from build123d import *

# Parameters (mm, degrees)
BOSS_EXTRUDE1_DEPTH             = 17.5
BOSS_EXTRUDE1_DEPTH_BACK        = 17.5
BOSS_EXTRUDE2_DEPTH             = 16
BOSS_EXTRUDE2_DEPTH_BACK        = 16
SKETCH1_3_R                     = 1
SKETCH1_3_W                     = 27.956190476
SKETCH1_3_H                     = 2.76
BOSS_EXTRUDE3_DEPTH             = 18.625
BOSS_EXTRUDE3_DEPTH_BACK        = 18.625
TAP_DRILL_FOR_2_HELICOIL1_D     = 2.38252
TAP_DRILL_FOR_2_HELICOIL1_DEPTH = 5
TAP_DRILL_FOR_2_HELICOIL1_TIP   = 0.715781221
SKETCH6_R                       = 9.6
SKETCH6_R_2                     = 4
CUT_EXTRUDE1_DEPTH              = 0.5


with BuildPart() as part:
    # Sketch1 → Boss-Extrude1 (new, two sides: drawn at the far end of the back side and taken through both)
    with BuildSketch(Plane.XY.offset(-BOSS_EXTRUDE1_DEPTH_BACK)):
        with BuildLine():
            Line((22.61, 0), (-0.726109068, 0))
            ThreePointArc((-0.726109068, 0), (-1.941229139, -5.326939839), (-5.346190476, -9.6))
            Line((-5.346190476, -9.6), (22.61, -9.6))
            Line((22.61, -9.6), (22.61, 0))
        make_face()
        with BuildLine():
            Line((22.61, 9.6), (-5.346190476, 9.6))
            ThreePointArc((-5.346190476, 9.6), (-1.941229139, 5.326939839), (-0.726109068, 0))
            Line((-0.726109068, 0), (22.61, 0))
            Line((22.61, 0), (22.61, 9.6))
        make_face()
    extrude(amount=BOSS_EXTRUDE1_DEPTH + BOSS_EXTRUDE1_DEPTH_BACK)

    # Sketch1<3> → Boss-Extrude2 (add, two sides: drawn at the far end of the back side and taken through both)
    # profile 1 of 7: a face of its own
    with BuildSketch(Plane.XY.offset(-BOSS_EXTRUDE2_DEPTH_BACK)):
        with BuildLine():
            ThreePointArc((-5.346190476, -9.6), (-1.941229139, -5.326939839), (-0.726109068, 0))
            Line((-0.726109068, 0), (-3.41, 0))
            ThreePointArc((-3.41, 0), (-13.01, -9.6), (-22.61, 0))
            Line((-22.61, 0), (-22.61, -12.36))
            Line((-22.61, -12.36), (-5.346190476, -12.36))
            Line((-5.346190476, -12.36), (-5.346190476, -9.6))
        make_face()
    # profile 2 of 7: a face of its own
    with BuildSketch(Plane.XY.offset(-BOSS_EXTRUDE2_DEPTH_BACK)):
        with BuildLine():
            ThreePointArc((-22.61, 0), (-13.01, -9.6), (-3.41, 0))
            Line((-3.41, 0), (-22.61, 0))
        make_face()
    # profile 3 of 7: a face of its own
    with BuildSketch(Plane.XY.offset(-BOSS_EXTRUDE2_DEPTH_BACK)):
        with BuildLine():
            Line((-22.61, 0), (-3.41, 0))
            ThreePointArc((-3.41, 0), (-13.01, 9.6), (-22.61, 0))
        make_face()
    # profile 4 of 7: a face of its own
    with BuildSketch(Plane.XY.offset(-BOSS_EXTRUDE2_DEPTH_BACK)):
        with BuildLine():
            ThreePointArc((-22.61, 0), (-13.01, -9.6), (-3.41, 0))
            Line((-3.41, 0), (-22.61, 0))
        make_face()
    # profile 5 of 7: a face of its own
    with BuildSketch(Plane.XY.offset(-BOSS_EXTRUDE2_DEPTH_BACK)):
        with BuildLine():
            Line((-22.61, 0), (-3.41, 0))
            ThreePointArc((-3.41, 0), (-13.01, 9.6), (-22.61, 0))
        make_face()
    # profile 6 of 7: a face of its own
    with BuildSketch(Plane.XY.offset(-BOSS_EXTRUDE2_DEPTH_BACK)):
        with BuildLine():
            ThreePointArc((-0.726109068, 0), (-1.941229139, 5.326939839), (-5.346190476, 9.6))
            Line((-5.346190476, 9.6), (22.61, 9.6))
            Line((22.61, 9.6), (22.61, 12.36))
            Line((22.61, 12.36), (-22.61, 12.36))
            Line((-22.61, 12.36), (-22.61, 0))
            ThreePointArc((-22.61, 0), (-13.01, 9.6), (-3.41, 0))
            Line((-3.41, 0), (-0.726109068, 0))
        make_face()
        with Locations((-4.2, 10.98)):
            Circle(SKETCH1_3_R, mode=Mode.SUBTRACT)
        with Locations((16.5, 10.98)):
            Circle(SKETCH1_3_R, mode=Mode.SUBTRACT)
    # profile 7 of 7: a face of its own
    with BuildSketch(Plane.XY.offset(-BOSS_EXTRUDE2_DEPTH_BACK)):
        with Locations((8.631904762, -10.98)):
            Rectangle(SKETCH1_3_W, SKETCH1_3_H)
        with Locations((-4.2, -10.98)):
            Circle(SKETCH1_3_R, mode=Mode.SUBTRACT)
        with Locations((16.5, -10.98)):
            Circle(SKETCH1_3_R, mode=Mode.SUBTRACT)
    extrude(amount=BOSS_EXTRUDE2_DEPTH + BOSS_EXTRUDE2_DEPTH_BACK)

    # Sketch1<4> → Boss-Extrude3 (add, two sides: drawn at the far end of the back side and taken through both)
    with BuildSketch(Plane.XY.offset(-BOSS_EXTRUDE3_DEPTH_BACK)):
        with BuildLine():
            ThreePointArc((-22.61, 0), (-13.01, -9.6), (-3.41, 0))
            Line((-3.41, 0), (-22.61, 0))
        make_face()
        with BuildLine():
            Line((-22.61, 0), (-3.41, 0))
            ThreePointArc((-3.41, 0), (-13.01, 9.6), (-22.61, 0))
        make_face()
    extrude(amount=BOSS_EXTRUDE3_DEPTH + BOSS_EXTRUDE3_DEPTH_BACK)

    # Tap Drill for #2 Helicoil1
    with Locations(Plane.XY.offset(18.625)):
        with Locations((-13.01, 6.148263222), (-6.861736778, 0), (-13.01, -6.148263222), (-19.158263222, 0)):
            Hole(TAP_DRILL_FOR_2_HELICOIL1_D / 2, depth=TAP_DRILL_FOR_2_HELICOIL1_DEPTH)
            with Locations((0, 0, -(TAP_DRILL_FOR_2_HELICOIL1_DEPTH + TAP_DRILL_FOR_2_HELICOIL1_TIP / 2))):  # 118° drill point
                Cone(0, TAP_DRILL_FOR_2_HELICOIL1_D / 2, TAP_DRILL_FOR_2_HELICOIL1_TIP, mode=Mode.SUBTRACT)

    # Sketch6 → Cut-Extrude1 (cut)
    with BuildSketch(Plane.XY.offset(16)):
        with Locations((-13.01, 0)):
            Circle(SKETCH6_R)
        with Locations((-13.01, 0)):
            Circle(SKETCH6_R_2, mode=Mode.SUBTRACT)
    extrude(amount=CUT_EXTRUDE1_DEPTH, mode=Mode.SUBTRACT)


solid = part.part
The listing builds one solid part. Answer for the finished solid, in the listing's coordinates (mm). A direction names the side the tool comes from. Give positions to 0.01 mm unless a question says otherwise; leave off trailing zeros. Write each loop counter-clockwise with the first axis right and the second up, starting at its lowest first coordinate (ties: lowest second). Pieces come first, ordered by that corner, then holes.
1) For a pull along Y with two mould halves and no side action, classify faces 1 (the face through (8, 0, 17.5)), 2 (the face through (0, -12.36, 0)), 3 (the face through (-13.65, 7.153, 17.548)) as pulls with the +Y half, pulls with the -Y half, needs draft (parallel to the pull), parting line crosses it, or undercut.
2) A tool of negligible diameter and unlimited length cuts with its end or side. For faces 4 (the face through (-7.998, 0.358, 17.548)), 5 (the face through (-13, 0, 18.625)), 6 (the face through (9, 9.6, 17)), from which of +Z, -Z, +X, -X, +Y, -Y can it reach the whole face along a straight path? Write none if from no direction.
3) Given P1, Ø1.2, axis at x = -4.2, y = -10.98, coming from the -Z side; P2, Ø9.5, axis at x = 9.5, y = -1.5, coming from the -Z side; P3, Ø3, axis at x = 16.5, y = -10.98, coming from the +Z side; P4, Ø1.9, axis at x = -13.01, y = 6.15, coming from the +Z side, each flat-ended and moving along its own axis, determine where each tip first touches the part or whether it passes through.
4) Section A-A (x = 16.5) is taken. Write down the section's boundary in (y, z), and give its area (3 significant figures).
5) Section C-C (x = 10) is taken. Write down the section's boundary in (y, z).
6) Section D-D (y = 9) is taken. Write down the section's boundary in (x, z) (3 decimals), and give its area (3 significant figures).
7) Section B-B (y = -8) is taken. Write down the section's boundary in (x, z) (3 decimals).
8) Find the intervals of material crossed by L1, parallel to Y at x = -13.01, z = 14.85; L2, parallel to Y at x = 16.5, z = -5.5; L3, parallel to X at y = 0, z = 14.2, in increasing order.
Response:
1. face 1: needs draft
1. face 2: pulls with the -Y half
1. face 3: undercut
2. face 4: +Z
2. face 5: +Z, +X, -X, +Y, -Y
2. face 6: +Z, +X, -X, +Y
3. P1: passes through
3. P2: stops at z = -17.5
3. P3: stops at z = 17.5
3. P4: stops at z = 13.48
4. outline: (-12.36, -16) - (-11.98, -16) - (-11.98, 16) - (-12.36, 16) - close; (-9.98, -16) - (-9.6, -16) - (-9.6, -17.5) - (9.6, -17.5) - (9.6, -16) - (9.98, -16) - (9.98, 16) - (9.6, 16) - (9.6, 17.5) - (-9.6, 17.5) - (-9.6, 16) - (-9.98, 16) - close; (11.98, -16) - (12.36, -16) - (12.36, 16) - (11.98, 16) - close
4. area: 721 mm2
5. outline: (-12.36, -16) - (-9.6, -16) - (-9.6, -17.5) - (9.6, -17.5) - (9.6, -16) - (12.36, -16) - (12.36, 16) - (9.6, 16) - (9.6, 17.5) - (-9.6, 17.5) - (-9.6, 16) - (-12.36, 16) - close
6. outline: (-22.61, -16) - (-16.351, -16) - (-16.351, -18.625) - (-9.669, -18.625) - (-9.669, -16) - (-4.65, -16) - (-4.65, -17.5) - (22.61, -17.5) - (22.61, 17.5) - (-4.65, 17.5) - (-4.65, 16) - (-22.61, 16) - close; (-16.351, 16.5) - (-9.669, 16.5) - (-9.669, 18.625) - (-16.351, 18.625) - close
6. area: 1,560 mm2
7. outline: (-22.61, -16) - (-18.317, -16) - (-18.317, -18.625) - (-7.703, -18.625) - (-7.703, -16) - (-3.688, -16) - (-3.688, -17.5) - (22.61, -17.5) - (22.61, 17.5) - (-3.688, 17.5) - (-3.688, 16) - (-22.61, 16) - close; (-18.317, 16.5) - (-7.703, 16.5) - (-7.703, 18.625) - (-18.317, 18.625) - close
8. L1: y = -12.36 to -7.34, -4.96 to 4.96, 7.34 to 12.36
8. L2: y = -12.36 to -11.98, -9.98 to 9.98, 11.98 to 12.36
8. L3: x = -22.61 to -20.35, -17.97 to -8.05, -5.67 to 22.61
